from build123d import *

# Parameters (mm, degrees)
BOSS_EXTRUDE1_START = -216
SKETCH3_W           = 13
SKETCH3_H           = 5
BOSS_EXTRUDE1_DEPTH = 5
BOSS_EXTRUDE2_START = -211
SKETCH3_4_W         = 5
SKETCH3_4_H         = 5
BOSS_EXTRUDE2_DEPTH = 30
BOSS_EXTRUDE3_START = -181
SKETCH3_5_W         = 50
SKETCH3_5_H         = 220
BOSS_EXTRUDE3_DEPTH = 5
BOSS_EXTRUDE4_START = -176
SKETCH3_6_W         = 5
SKETCH3_6_H         = 5
SKETCH3_6_W_2       = 50
BOSS_EXTRUDE4_DEPTH = 176
SKETCH6_R           = 8.5
CUT_EXTRUDE1_DEPTH  = 371.885427053


with BuildPart() as part:
    # Sketch3 → Boss-Extrude1 (new body)
    with BuildSketch(Plane(origin=(0, 0, 0), x_dir=(0, 0, -1), z_dir=(1, 0, 0)).offset(BOSS_EXTRUDE1_START)):
        with BuildLine():
            Line((-30, 0), (-30, 300))
            Line((-30, 300), (30, 300))
            Line((30, 300), (30, 0))
            ThreePointArc((30, 0), (0, -30), (-30, 0))
        make_face()
        with Locations((0, 48)):
            Rectangle(SKETCH3_W, SKETCH3_H, mode=Mode.SUBTRACT)
    extrude(amount=BOSS_EXTRUDE1_DEPTH)

    # Sketch3<4> → Boss-Extrude2 (add)
    with BuildSketch(Plane(origin=(0, 0, 0), x_dir=(0, 0, -1), z_dir=(1, 0, 0)).offset(BOSS_EXTRUDE2_START)):
        Polygon((-30, 300), (-30, 75), (-25, 75), (-25, 295), (25, 295), (25, 75), (30, 75), (30, 300), align=None)
        with BuildLine():
            Line((-30, 70), (-30, 0))
            ThreePointArc((-30, 0), (0, -30), (30, 0))
            Line((30, 0), (30, 70))
            Line((30, 70), (25, 70))
            Line((25, 70), (25, 0))
            ThreePointArc((25, 0), (0, -25), (-25, 0))
            Line((-25, 0), (-25, 70))
            Line((-25, 70), (-30, 70))
        make_face()
        with Locations((-27.5, 72.5)):
            Rectangle(SKETCH3_4_W, SKETCH3_4_H)
        with Locations((27.5, 72.5)):
            Rectangle(SKETCH3_4_W, SKETCH3_4_H)
    extrude(amount=BOSS_EXTRUDE2_DEPTH)

    # Sketch3<5> → Boss-Extrude3 (add)
    with BuildSketch(Plane(origin=(0, 0, 0), x_dir=(0, 0, -1), z_dir=(1, 0, 0)).offset(BOSS_EXTRUDE3_START)):
        with BuildLine():
            ThreePointArc((-30, 0), (0, -30), (30, 0))
            Line((30, 0), (30, 300))
            Line((30, 300), (-30, 300))
            Line((-30, 300), (-30, 0))
        make_face()
        with Locations((0, 185)):
            Rectangle(SKETCH3_5_W, SKETCH3_5_H, mode=Mode.SUBTRACT)
    extrude(amount=BOSS_EXTRUDE3_DEPTH)

    # Sketch3<6> → Boss-Extrude4 (add)
    with BuildSketch(Plane(origin=(0, 0, 0), x_dir=(0, 0, -1), z_dir=(1, 0, 0)).offset(BOSS_EXTRUDE4_START)):
        Polygon((-30, 300), (-30, 75), (-25, 75), (-25, 295), (25, 295), (25, 75), (30, 75), (30, 300), align=None)
        with Locations((-27.5, 72.5)):
            Rectangle(SKETCH3_6_W, SKETCH3_6_H)
        with Locations((0, 72.5)):
            Rectangle(SKETCH3_6_W_2, SKETCH3_6_H)
        with Locations((27.5, 72.5)):
            Rectangle(SKETCH3_6_W, SKETCH3_6_H)
    extrude(amount=BOSS_EXTRUDE4_DEPTH)

    # Sketch6 → Cut-Extrude1 (cut, through all)
    with BuildSketch(Plane(origin=(0, 0, 0), x_dir=(0, 0, -1), z_dir=(1, 0, 0))):
        Circle(SKETCH6_R)
    extrude(amount=-CUT_EXTRUDE1_DEPTH, mode=Mode.SUBTRACT)

    # Mirror5: part across plane


with BuildPart() as part_1:
    add(part.part)
    add(part.part.mirror(Plane(origin=(0, 0, 0), x_dir=(0, 0, 1), z_dir=(1, 0, 0))))


solid = part_1.part
CAD build for the part. Positions are in the model's coordinates, mm. A direction names the side the tool comes from. Round coordinates to 2 decimals unless told otherwise and drop trailing zeros. Order: outer loops, then holes, each group sorted by start corner. A loop starts at its lowest first (then second) coordinate and runs counter-clockwise, first axis right, second up. Notation, with made-up numbers: (30.25, 22) -> (69.25, 22) arc R21 ccw to (69.25, 44) -> close; hole circle Ø11 at (-2.5, 8.5). An arc over 180 degrees is marked (long way). Write each question's results on one line, items separated by ' | '.
1. Wall check: line 1 along X through (y, z) = (4, 11); line 2 along Y through (x, z) = (177.95, 0); line 3 along Z through (x, y) = (33, 115). Give the ranges that are in metal, low to high. Write a range as [from, to].
Findings below:
line 1: x = [-216, -211], [-181, -176], [176, 181], [211, 216] | line 2: y = [-30, -8.5], [8.5, 75], [295, 300] | line 3: z = [-30, -25], [25, 30]
2. Cut at A-A (y = 29). Give the cut face in (x, z).
Findings below:
outline: (-216, -30) -> (-176, -30) -> (-176, 30) -> (-216, 30) -> close; (176, -30) -> (216, -30) -> (216, 30) -> (176, 30) -> close; hole (-211, -25) -> (-181, -25) -> (-181, 25) -> (-211, 25) -> close; hole (181, -25) -> (211, -25) -> (211, 25) -> (181, 25) -> close
3. 3-axis set-ups, long thin cutter, end or side, ignore diameter. For faces 5 (the face through (-176, 21, 0)), 6 (the face through (196.28, -29.993, 0.66)), 7 (the face through (181, 26, 0)): which of +Z, -Z, +X, -X, +Y, -Y reach the whole face in a straight line?
Findings below:
face 5: +Z, -Z, -Y | face 6: +X, -X, -Y | face 7: none
4. Flat gauge pins, fed straight in: P1, Ø25, axis at x = 37, z = -9, coming from the -Y side; P2, Ø2.5, axis at x = -212.5, z = -1, coming from the -Y side; P3, Ø19.5, axis at y = 0, z = 0, coming from the -X side. Where does each tip first touch, or does it go through?
Findings below:
P1: stops at y = 70 | P2: stops at y = -30 | P3: stops at x = -216
5. Pull direction X, two halves, no side cores. Call faces 1 (the face through (-216, 137, 0)), 2 (the face through (3, 185, 30)), 3 (the face through (3, 75, 0)), 4 (the face through (-181, 26, 0)): pulls with the +X half, pulls with the -X half, needs draft (parallel to the pull), parting line crosses it, or undercut.
Findings below:
face 1: pulls with the -X half | face 2: needs draft | face 3: undercut | face 4: undercut
6. Cut at D-D (y = 101.5). Give the cut face in (x, z).
Findings below:
outline: (-216, -30) -> (216, -30) -> (216, 30) -> (-216, 30) -> close; hole (-211, -25) -> (211, -25) -> (211, 25) -> (-211, 25) -> close
7. Cut at B-B (x = -68). Give the cut face in (y, z), plus the area to 3 significant figures.
Findings below:
outline: (70, -30) -> (300, -30) -> (300, 30) -> (70, 30) -> close; hole (75, -25) -> (295, -25) -> (295, 25) -> (75, 25) -> close | area: 2,800 mm²
8. Cut at C-C (z = 0). Count the separate pieces of the cut face and the enclosed holes in it, plus the area to 3 significant figures.
Findings below:
separate pieces: 6 | enclosed holes: 0 | area: 8,130 mm²
